from build123d import *

# Parameters (mm, degrees)
BOSS_EXTRUDE8_DEPTH = 6.35


with BuildPart() as part:
    # Sketch1 → Boss-Extrude8 (new body)
    with BuildSketch(Plane(origin=(0, 0, -3683), x_dir=(-1, 0, 0), z_dir=(0, 0, -1))):
        with BuildLine():
            Line((12.7, 4.064), (3.556, 4.064))
            ThreePointArc((3.556, 4.064), (3.106987194, 4.249987194), (2.921, 4.699))
            Line((2.921, 4.699), (2.921, 6.223))
            ThreePointArc((2.921, 6.223), (3.106987194, 6.672012806), (3.556, 6.858))
            Line((3.556, 6.858), (6.376363549, 6.858))
            Line((6.376363549, 6.858), (6.376363549, 7.365999958))
            Line((6.376363549, 7.365999958), (2.54, 11.938))
            Line((2.54, 11.938), (-2.54, 11.938))
            Line((-2.54, 11.938), (-6.376363549, 7.365999958))
            Line((-6.376363549, 7.365999958), (-6.376363549, 6.858))
            Line((-6.376363549, 6.858), (-3.556, 6.858))
            ThreePointArc((-3.556, 6.858), (-3.106987194, 6.672012806), (-2.921, 6.223))
            Line((-2.921, 6.223), (-2.921, 4.699))
            ThreePointArc((-2.921, 4.699), (-3.106987194, 4.249987194), (-3.556, 4.064))
            Line((-3.556, 4.064), (-12.7, 4.064))
            Line((-12.7, 4.064), (-16.764, 0))
            Line((-16.764, 0), (-12.7, 0))
            Line((-12.7, 0), (12.7, 0))
            Line((12.7, 0), (16.764, 0))
            Line((16.764, 0), (12.7, 4.064))
        make_face()
    extrude(amount=BOSS_EXTRUDE8_DEPTH)


solid = part.part
Could you check a few things on this model? Use its own coordinates, in mm. A direction names the side the tool comes from. Give positions to 0.01 mm unless a question says otherwise; leave off trailing zeros. Write each loop counter-clockwise with the first axis right and the second up, starting at its lowest first coordinate (ties: lowest second). Pieces come first, ordered by that corner, then holes. Notation, with made-up numbers: (38.25, 16) -> (48.25, 16) arc R12 cw to (48.25, 35) -> close; hole circle Ø5 at (-1, -26). An arc over 180 degrees is marked (long way). Write each question's results on one line, items separated by ' | '. Start each with the question number.
Q1. I need wall thicknesses on probe 1 along Y at (x, z) = (11, -3687.5); probe 2 along X at (y, z) = (5.5, -3683.75); probe 3 along Y at (x, z) = (4, -3683.5). Which ranges of each line are inside material? Lowest first, please.
Q2. We'd pull the mould along Y, two halves only. Please class faces 1 (the face through (8, 4.064, -3686)), 2 (the face through (0, 11.938, -3686)), 3 (the face through (2.921, 5, -3686)), 4 (the face through (0, 5, -3689.35)): +Y half, -Y half, draft (parallel to the pull), parting line (faces both ways), or undercut.
Q3. Suppose I cut it at D-D, the plane y = 1.5. List the corners of the cut face in (x, z) for me.
Q4. Suppose I cut it at A-A, the plane x = 5.5. List the corners of the cut face in (y, z) for me.
Q5. Suppose I cut it at B-B, the plane z = -3684. List the corners of the cut face in (x, y) for me (3 decimals).
Q6. I'm going to push flat-ended pins straight in: pin 1 Ø1.5 at (y, z) = (10.5, -3685) entering from -X; pin 2 Ø1.7 at (y, z) = (5.5, -3687) entering from +X; pin 3 Ø1.5 at (y, z) = (9, -3686.5) entering from -X. Where does each tip first touch, or does it pass through?
Q7. Suppose I cut it at C-C, the plane x = -4.5. List the corners of the cut face in (y, z) for me, and give its area (3 significant figures).
Q8. Which directions (+Z, -Z, +X, -X, +Y, -Y) give clear straight access to the entire face, cutting with the end or side of a thin tool? Please do faces 5 (the face through (-4.5, 9.6, -3686.1)), 6 (the face through (-2.921, 5, -3686)), 7 (the face through (5, 6.858, -3686)).
Outcome:
1) probe 1: 0 to 4.06 | probe 2: -2.92 to 2.92 | probe 3: 0 to 4.06, 6.86 to 10.2
2) face 1: undercut | face 2: +Y half | face 3: undercut | face 4: draft
3) outline: (-15.26, -3689.35) -> (15.26, -3689.35) -> (15.26, -3683) -> (-15.26, -3683) -> close
4) outline: (0, -3689.35) -> (4.06, -3689.35) -> (4.06, -3683) -> (0, -3683) -> close; (6.86, -3689.35) -> (8.41, -3689.35) -> (8.41, -3683) -> (6.86, -3683) -> close
5) outline: (-16.764, 0) -> (16.764, 0) -> (12.7, 4.064) -> (3.556, 4.064) arc R0.635 cw to (2.921, 4.699) -> (2.921, 6.223) arc R0.635 cw to (3.556, 6.858) -> (6.376, 6.858) -> (6.376, 7.366) -> (2.54, 11.938) -> (-2.54, 11.938) -> (-6.376, 7.366) -> (-6.376, 6.858) -> (-3.556, 6.858) arc R0.635 cw to (-2.921, 6.223) -> (-2.921, 4.699) arc R0.635 cw to (-3.556, 4.064) -> (-12.7, 4.064) -> close
6) pin 1: x = -4.38 | pin 2: x = 2.93 | pin 3: x = -5.63
7) outline: (0, -3689.35) -> (4.06, -3689.35) -> (4.06, -3683) -> (0, -3683) -> close; (6.86, -3689.35) -> (9.6, -3689.35) -> (9.6, -3683) -> (6.86, -3683) -> close | area: 43.2 mm2
8) face 5: +Z, -Z, -X, +Y | face 6: +Z, -Z, -X | face 7: +Z, -Z, +X
